```python
from build123d import *

# Parameters (mm, degrees)
F0_W      = 15
F0_H      = 15
F1_DEPTH  = 22.5
F2_W      = 50
F2_H      = 22
F3_DEPTH  = 12.5
F5_DEPTH  = 12.7
F6_R      = 10
F7_DEPTH  = 3
F8_R      = 2
F9_DEPTH  = 4
F10_R     = 1.27
F11_R     = 3.941379
F12_DEPTH = 8
F13_R     = 2.54


with BuildPart() as f1:
    # F0 (on Front) → F1 (new body, symmetric)
    with BuildSketch(Plane.XZ):
        Rectangle(F0_W, F0_H)
    extrude(amount=F1_DEPTH, both=True)

    # F2 (on Right) → F3 (join, symmetric)
    with BuildSketch(Plane.YZ):
        with Locations((0, 18.5)):
            Rectangle(F2_W, F2_H)
    extrude(amount=F3_DEPTH, both=True)

    # F4 (on Right) → F5 (cut, symmetric)
    with BuildSketch(Plane.YZ):
        with BuildLine():
            Line((-25, 29.5), (-25, 22.5))
            ThreePointArc((-25, 22.5), (-20.050253, 24.550253), (-18, 29.5))
            Line((-18, 29.5), (-25, 29.5))
        make_face()
        with BuildLine():
            ThreePointArc((18, 29.5), (20.050253, 24.550253), (25, 22.5))
            Line((25, 22.5), (25, 29.5))
            Line((25, 29.5), (18, 29.5))
        make_face()
    extrude(amount=F5_DEPTH, both=True, mode=Mode.SUBTRACT)

    # F6 (on face) → F7 (join)
    with BuildSketch(Plane.YZ.offset(7.5)):
        with Locations((12.5, -5.5)):
            Circle(F6_R)
        with Locations((-12.5, -5.5)):
            Circle(F6_R)
    extrude(amount=F7_DEPTH)

    # F8 (on face) → F9 (join)
    with BuildSketch(Plane.YZ.offset(10.5)):
        with Locations((12.5, -5.5)):
            Circle(F8_R)
    extrude(amount=F9_DEPTH)

    # F10
    f10_edges = [f1.edges().sort_by_distance(p)[0] for p in [
        (14.5, 10.5, -5.5),
    ]]
    fillet(f10_edges, radius=F10_R)

    # F11 (on face) → F12 (join)
    with BuildSketch(Plane(origin=(0, 22.5, 0), x_dir=(-1, 0, 0), z_dir=(0, 1, 0))):
        Circle(F11_R)
    extrude(amount=F12_DEPTH)

    # F13
    f13_edges = [f1.edges().sort_by_distance(p)[0] for p in [
        (3.941379, 30.5, 0),
    ]]
    fillet(f13_edges, radius=F13_R)

    # F14: F1 across plane


with BuildPart() as f1_1:
    add(f1.part)
    add(f1.part.mirror(Plane.YZ))

    # F15: F1 across plane


with BuildPart() as f1_2:
    add(f1_1.part)
    add(f1_1.part.mirror(Plane.XZ))


solid = f1_2.part
```
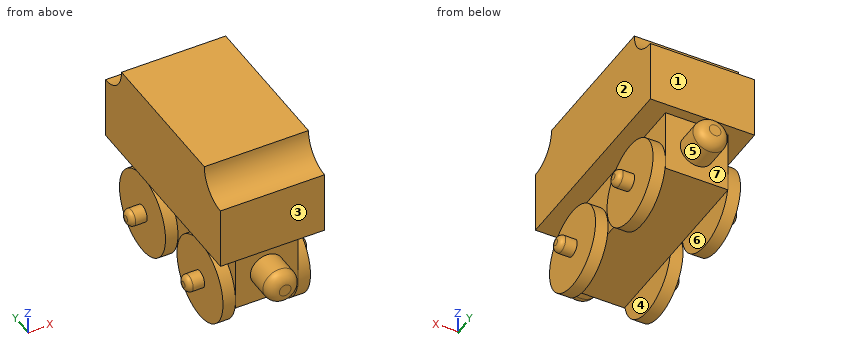
Could you check a few things on this model? Use its own coordinates, in mm. Face numbers are marked on the shaded views. A direction names the side the tool comes from. Round coordinates to 2 decimals unless told otherwise and drop trailing zeros. Write each loop counter-clockwise with the first axis right and the second up, starting at its lowest first coordinate (ties: lowest second). Pieces come first, ordered by that corner, then holes. Notation, with made-up numbers: M 30,35.25 L 45,35.25 A11 cw 45,50.25 Z; hole C 68.5,-6 d6. An arc over 180 degrees is marked long. Answer in a Markdown table with one row per item. Add a question column.
Q1. If we mould it in two halves opening along X, with no side actions, what happens to the marked faces 4, 5, 6 and 7? For each: +X half, -X half, draft (parallel to the pull), parting line (faces both ways), or undercut.
Q2. Imagine slicing it at D-D (x = 11.25). Please give me the cut outline in (y, z), then the cut area to 3 significant figures.
Q3. Imagine slicing it at A-A (x = -9). Please give me the cut outline in (y, z).
Q4. Imagine slicing it at B-B (z = -8.5). Please give me the cut outline in (x, y), then the cut area to 3 significant figures.
Q5. Imagine slicing it at C-C (y = -1). Please give me the cut outline in (x, z), then the cut area to 3 significant figures.
Q6. On a 3-axis mill with a long thin cutter (end or side, diameter ignored), from which of +Z, -Z, +X, -X, +Y, -Y can I reach the whole of each face in a straight line? I mean the marked faces 1, 2 and 3. Say none if no direction works.
Q7. Will these pins go through, and if not, where does the flat tip stop? pin 1 Ø4.5 at (x, z) = (-2, 17.5) entering from -Y; pin 2 Ø4.5 at (y, z) = (-3.5, 3.5) entering from +X; pin 3 Ø4.5 at (y, z) = (-5, -2) entering from -X.
Q8. If I drill on line 1 (X direction, y = 22, z = 1.5); line 2 (X direction, y = 8, z = 10); line 3 (Y direction, x = -7.5, z = 18), over which ranges is the centre line in solid material (lowest first)? Write a range as from..to.
Values:
| question | item | result |
|---|---|---|
| 1 | face 4 | undercut |
| 1 | face 5 | parting line |
| 1 | face 6 | undercut |
| 1 | face 7 | draft |
| 2 | outline | M -25,7.5 L 25,7.5 L 25,22.5 A7 cw 18,29.5 L -18,29.5 A7 cw -25,22.5 Z; C -12.5,-5.5 d4; C 12.5,-5.5 d4 |
| 2 | area | 1,050 mm^2 |
| 3 | outline | M -25,7.5 L 25,7.5 L 25,22.5 A7 cw 18,29.5 L -18,29.5 A7 cw -25,22.5 Z; C -12.5,-5.5 d20; C 12.5,-5.5 d20 |
| 4 | outline | M -10.5,-22.04 L -7.5,-22.04 L -7.5,-2.96 L -10.5,-2.96 Z; M -10.5,2.96 L -7.5,2.96 L -7.5,22.04 L -10.5,22.04 Z; M 7.5,-22.04 L 10.5,-22.04 L 10.5,-2.96 L 7.5,-2.96 Z; M 7.5,2.96 L 10.5,2.96 L 10.5,22.04 L 7.5,22.04 Z |
| 4 | area | 229 mm^2 |
| 5 | outline | M -12.5,7.5 L -7.5,7.5 L -7.5,-7.5 L 7.5,-7.5 L 7.5,7.5 L 12.5,7.5 L 12.5,29.5 L -12.5,29.5 Z |
| 5 | area | 775 mm^2 |
| 6 | face 1 | +Z, +X, -X, +Y |
| 6 | face 2 | +Z, +X, +Y, -Y |
| 6 | face 3 | +Z, +X, -X, -Y |
| 7 | pin 1 | y = -25 |
| 7 | pin 2 | x = 7.5 |
| 7 | pin 3 | x = -10.5 |
| 8 | line 1 | -7.5..7.5 |
| 8 | line 2 | -12.5..12.5 |
| 8 | line 3 | -25..25 |
